```python
from build123d import *

# Parameters (mm, degrees)
F2_SIZE = 2
F3_SIZE = 0.75
F4_SIZE = 0.5
F5_R    = 0.5


# Not quite as in the source:
# - a fillet or chamfer that OpenCascade refuses, or shapes differently, is made with other operations: its cross-section is extruded or revolved along the edge and cut away or added


with BuildPart() as f1:
    # F0 (on Front) → F1 (revolve)
    with BuildSketch(Plane.XZ):
        Polygon((17.025, 33.05), (17.025, 0), (40, 0), (40, 2), (35, 2), (35, 8.05), (40, 8.05), (40, 11.05), (23.25, 11.05), (23.25, 15.05), (19.059525, 15.05), (19.059525, 33.05), align=None)
    revolve(axis=Axis((0, 0, 13.9434672892), (0, 0, 1)))

    # F2
    f2_edges = [f1.edges().sort_by_distance(p)[0] for p in [
        (-17.025, 0, 0),
    ]]
    chamfer(f2_edges, length=F2_SIZE)

    # F3
    f3_edges = [f1.edges().sort_by_distance(p)[0] for p in [
        (-17.025, 0, 33.05),
        (-19.059525, 0, 33.05),
    ]]
    chamfer(f3_edges, length=F3_SIZE)

    # F4
    f4_edges = [f1.edges().sort_by_distance(p)[0] for p in [
        (-23.25, 0, 15.05),
        (-40, 0, 8.05),
        (-40, 0, 2),
    ]]
    chamfer(f4_edges, length=F4_SIZE)

    # F5
    f5_edges = [f1.edges().sort_by_distance(p)[0] for p in [
        (-35, 0, 8.05),
        (-35, 0, 2),
        (-19.059525, 0, 15.05),
    ]]
    fillet(f5_edges, radius=F5_R)

    # F6: fillet of radius 5 on 1 edges, made by hand

    # F6_s1 → F6_t2 (revolve)
    with BuildSketch(Plane.XZ):
        with BuildLine():
            ThreePointArc((28.0196960071, 11.05), (25.0616561155, 12.0188711259), (23.25, 14.55))
            Line((23.25, 14.55), (23.1546060799, 14.52))
            ThreePointArc((23.1546060799, 14.52), (23.15, 12.8), (23.15, 11.05))
            Line((23.15, 11.05), (23.25, 10.95))
            Line((23.25, 10.95), (28.0196960071, 10.95))
            Line((28.0196960071, 10.95), (28.0196960071, 11.05))
        make_face()
    revolve(axis=Axis((0, 0, 11.05), (0, 0, 1)))


solid = f1.part
```
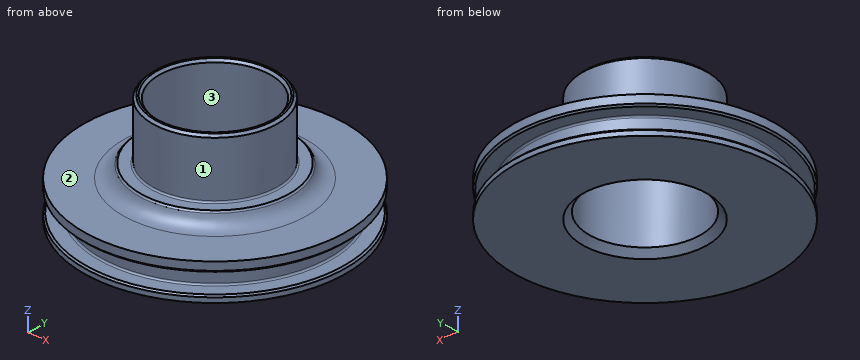
The listing builds one solid part. Answer for the finished solid, in the listing's coordinates (mm). Face numbers are marked on the shaded views. Coordinates: 2 decimals unless noted, no trailing zeros. Write each loop counter-clockwise with the first axis right and the second up, starting at its lowest first coordinate (ties: lowest second). Pieces come first, ordered by that corner, then holes. Notation, with made-up numbers: M -8.5,-28 L 20.5,-28 A27 ccw 20.5,-9 Z; hole C 72.25,9 d5. An arc over 180 degrees is marked long. Use a Markdown table: item, result. Add a question column.
1. For a pull along X with two mould halves and no side action, classify the marked faces 1, 2 and 3 as +X half, -X half, draft (parallel to the pull), parting line (faces both ways), or undercut.
2. Given P1, Ø6, axis at y = 8, z = 6, coming from the +X side; P2, Ø4, axis at x = 12, z = 9, coming from the -Y side; P3, Ø1.5, axis at y = -31, z = 4, coming from the +X side; P4, Ø20.5, axis at x = 0, y = 0, coming from the +Z side, each flat-ended and moving along its own axis, determine where each tip first touches the part or whether it passes through.
3. Straight lines are drawn through the part: line 1 along Y through (x, z) = (0, 17) (3 decimals); line 2 along Y through (x, z) = (0, 9) (3 decimals); line 3 along Z through (x, y) = (-17, -31). For each, find the intervals that lie inside material, in ascending order. Write a range as [from, to].
4. Section A-A (z = 23) is taken. Give the vertices of the cut face in (x, y) (3 decimals), plus the area to 3 significant figures.
Data:
| question | item | result |
|---|---|---|
| 1 | face 1 | parting line |
| 1 | face 2 | draft |
| 1 | face 3 | undercut |
| 2 | P1 | stops at x = 39.48 |
| 2 | P2 | stops at y = -38.73 |
| 2 | P3 | stops at x = 17.61 |
| 2 | P4 | passes through |
| 3 | line 1 | y = [-19.06, -17.025], [17.025, 19.06] |
| 3 | line 2 | y = [-40, -17.025], [17.025, 40] |
| 3 | line 3 | z = [0, 2.02], [8.03, 11.05] |
| 4 | outline | C 0,0 d38.119; hole C 0,0 d34.05 |
| 4 | area | 231 mm2 |
